Verification items for the finished model (mm, model axes). Round coordinates to 2 decimals unless told otherwise and drop trailing zeros. Write each loop counter-clockwise with the first axis right and the second up, starting at its lowest first coordinate (ties: lowest second). Pieces come first, ordered by that corner, then holes. Notation, with made-up numbers: M 84.25,-22 L 105.25,-22 A23 cw 105.25,-3 Z; hole C 56,50 d1. An arc over 180 degrees is marked long. Write each question's results on one line, items separated by ' | '.
from build123d import *

# Parameters (mm, degrees)
SKETCH_1_W          = 41
SKETCH_1_H          = 60
EXTRUDE_1_DEPTH     = 4
SKETCH_2_R          = 1.75
CUT_EXTRUDE_1_DEPTH = 37.554753453
FILLET_1_R          = 2
CHAMFER_2_SIZE      = 1
CHAMFER_1_SIZE      = 2
CHAMFER_3_SIZE      = 0.5


with BuildPart() as part:
    # Эскиз1 → Бобышка-Вытянуть1 (new body)
    with BuildSketch(Plane(origin=(0, 0, 0), x_dir=(1, 0, 0), z_dir=(0, 1, 0))):
        Rectangle(SKETCH_1_W, SKETCH_1_H)
    extrude(amount=EXTRUDE_1_DEPTH)

    # Эскиз2 → Вырез-Вытянуть1 (cut, through all)
    with BuildSketch(Plane(origin=(0, 4, 0), x_dir=(1, 0, 0), z_dir=(0, 1, 0))):
        with Locations(Location((17, 25, 0), (0, 0, 270))):
            Circle(SKETCH_2_R)
        with Locations(Location((17, -25, 0), (0, 0, 90))):
            Circle(SKETCH_2_R)
        with Locations(Location((-17, -25, 0), (0, 0, 270))):
            Circle(SKETCH_2_R)
        with Locations(Location((-17, 25, 0), (0, 0, 90))):
            Circle(SKETCH_2_R)
    extrude(amount=-CUT_EXTRUDE_1_DEPTH, mode=Mode.SUBTRACT)

    # Скругление1
    fillet_1_edges = [part.edges().sort_by_distance(p)[0] for p in [
        (20.5, 2, 30),
        (-20.5, 2, 30),
        (-20.5, 2, -30),
        (20.5, 2, -30),
    ]]
    fillet(fillet_1_edges, radius=FILLET_1_R)

    # Фаска2
    chamfer_2_edges = [part.edges().sort_by_distance(p)[0] for p in [
        (0, 4, -30),
        (20.5, 4, 0),
        (-20.5, 4, 0),
        (0, 4, 30),
        (19.914213562, 4, 29.414213562),
        (-19.914213562, 4, 29.414213562),
        (-19.914213562, 4, -29.414213562),
        (19.914213562, 4, -29.414213562),
    ]]
    chamfer(chamfer_2_edges, length=CHAMFER_2_SIZE)

    # Фаска1
    # the kernel refuses this chamfer: 2 mm, written as the material it takes off along each edge
    with BuildSketch(Plane(origin=(-17, 4, -25), x_dir=(0, 0, -1), z_dir=(1, 0, 0))) as chamfer_1_piece_1:
        Polygon((1.75 + CHAMFER_1_SIZE, 0), (1.75, -CHAMFER_1_SIZE), (1.75, 0), align=None)
    revolve(axis=Axis((-17, 4, -25), (0, 1, 0)), mode=Mode.SUBTRACT)
    with BuildSketch(Plane(origin=(-17, 4, 25), x_dir=(0, 0, 1), z_dir=(-1, 0, 0))) as chamfer_1_piece_2:
        Polygon((1.75 + CHAMFER_1_SIZE, 0), (1.75, -CHAMFER_1_SIZE), (1.75, 0), align=None)
    revolve(axis=Axis((-17, 4, 25), (0, 1, 0)), mode=Mode.SUBTRACT)
    with BuildSketch(Plane(origin=(17, 4, 25), x_dir=(0, 0, -1), z_dir=(1, 0, 0))) as chamfer_1_piece_3:
        Polygon((1.75 + CHAMFER_1_SIZE, 0), (1.75, -CHAMFER_1_SIZE), (1.75, 0), align=None)
    revolve(axis=Axis((17, 4, 25), (0, 1, 0)), mode=Mode.SUBTRACT)
    with BuildSketch(Plane(origin=(17, 4, -25), x_dir=(0, 0, 1), z_dir=(-1, 0, 0))) as chamfer_1_piece_4:
        Polygon((1.75 + CHAMFER_1_SIZE, 0), (1.75, -CHAMFER_1_SIZE), (1.75, 0), align=None)
    revolve(axis=Axis((17, 4, -25), (0, 1, 0)), mode=Mode.SUBTRACT)

    # Фаска3
    chamfer_3_edges = [part.edges().sort_by_distance(p)[0] for p in [
        (-17, 0, -23.25),
        (-17, 0, 23.25),
        (17, 0, 26.75),
        (17, 0, -26.75),
        (0, 0, -30),
        (20.5, 0, 0),
        (0, 0, 30),
        (-20.5, 0, 0),
        (19.914213562, 0, 29.414213562),
        (-19.914213562, 0, 29.414213562),
        (-19.914213562, 0, -29.414213562),
        (19.914213562, 0, -29.414213562),
    ]]
    chamfer(chamfer_3_edges, length=CHAMFER_3_SIZE)


solid = part.part
1) Material ranges on line 1 (X direction, y = 1.5, z = 25); line 2 (Z direction, x = 16.5, y = 1.75); line 3 (X direction, y = 3.3, z = 26), recorded low to high. Write a range as [from, to].
Calculated:
line 1: x = [-20.5, -18.75], [-15.25, 15.25], [18.75, 20.5] | line 2: z = [-30, -26.68], [-23.32, 23.32], [26.68, 30] | line 3: x = [-20.2, -19.88], [-14.12, 14.12], [19.88, 20.2]
2) Sectioned sample at A-A, the plane x = -17. Record the cut outline in (y, z).
Calculated:
outline: M 0,-29.5 L 0.5,-30 L 3,-30 L 4,-29 L 4,-28.75 L 2,-26.75 L 0.5,-26.75 L 0,-27.25 Z; M 0,-22.75 L 0.5,-23.25 L 2,-23.25 L 4,-21.25 L 4,21.25 L 2,23.25 L 0.5,23.25 L 0,22.75 Z; M 0,27.25 L 0.5,26.75 L 2,26.75 L 4,28.75 L 4,29 L 3,30 L 0.5,30 L 0,29.5 Z
3) Draft check along X on faces 1 (the conical face through (19.5, 3.6, 28.98)), 2 (the cylindrical face through (15.82, 1.26, 26.29)), 3 (the cylindrical face through (-19.93, 1.77, 29.4)). Enter one of: pulls with the +X half, pulls with the -X half, needs draft (parallel to the pull), parting line crosses it, or undercut.
Calculated:
face 1: pulls with the +X half | face 2: undercut | face 3: pulls with the -X half
4) Depth check by flat-ended pin: P1, Ø4, axis at x = -17, z = -25, coming from the -Y side; P2, Ø4.5, axis at x = 17, z = 25, coming from the +Y side. Enter the tip coordinate at first touch or a pass-through.
Calculated:
P1: stops at y = 0.25 | P2: stops at y = 2.5
5) Sectioned sample at C-C, the plane z = -25. Record the cut outline in (x, y) (3 decimals), and give its area (3 significant figures).
Calculated:
outline: M -20.5,0.5 L -20,0 L -19.25,0 L -18.75,0.5 L -18.75,2 L -20.125,3.375 L -20.5,3 Z; M -15.25,0.5 L -14.75,0 L 14.75,0 L 15.25,0.5 L 15.25,2 L 13.25,4 L -13.25,4 L -15.25,2 Z; M 18.75,0.5 L 19.25,0 L 20,0 L 20.5,0.5 L 20.5,3 L 20.125,3.375 L 18.75,2 Z | area: 127 mm²
6) Sectioned sample at B-B, the plane y = 1.35. Record the cut outline in (x, z).
Calculated:
outline: M -20.5,-28 A2 ccw -18.5,-30 L 18.5,-30 A2 ccw 20.5,-28 L 20.5,28 A2 ccw 18.5,30 L -18.5,30 A2 ccw -20.5,28 Z; hole C -17,-25 d3.5; hole C -17,25 d3.5; hole C 17,-25 d3.5; hole C 17,25 d3.5
